```python
from build123d import *

# Parameters (mm, degrees)
SKETCH1_R           = 12.685
SKETCH1_R_2         = 3
BOSS_EXTRUDE1_DEPTH = 5
SKETCH2_R           = 6
SKETCH2_R_2         = 3
BOSS_EXTRUDE2_DEPTH = 9.25
SKETCH3_R           = 1.5
CUT_EXTRUDE1_DEPTH  = 12
SKETCH5_R           = 1.5
CUT_EXTRUDE3_DEPTH  = 21.183680289


with BuildPart() as part:
    # Sketch1 → Boss-Extrude1 (new body)
    with BuildSketch(Plane(origin=(0, 0, 0), x_dir=(1, 0, 0), z_dir=(0, 1, 0))):
        with Locations(Location((0, 0, 0), (0, 0, 270))):
            Circle(SKETCH1_R)
        with Locations(Location((0, 0, 0), (0, 0, 270))):
            Circle(SKETCH1_R_2, mode=Mode.SUBTRACT)
    extrude(amount=BOSS_EXTRUDE1_DEPTH)

    # Sketch2 → Boss-Extrude2 (add)
    with BuildSketch(Plane(origin=(0, 0, 0), x_dir=(1, 0, 0), z_dir=(0, 1, 0))):
        with Locations(Location((0, 0, 0), (0, 0, 270))):
            Circle(SKETCH2_R)
        with Locations(Location((0, 0, 0), (0, 0, 270))):
            Circle(SKETCH2_R_2, mode=Mode.SUBTRACT)
    extrude(amount=BOSS_EXTRUDE2_DEPTH)

    # Sketch3 → Cut-Extrude1 (cut)
    with BuildSketch(Plane(origin=(0, 0, 0), x_dir=(1, 0, 0), z_dir=(0, 1, 0))):
        with Locations(Location((0, 10, 0), (0, 0, 270))):
            Circle(SKETCH3_R)
        with Locations(Location((8.660254038, 5, 0), (0, 0, 270))):
            Circle(SKETCH3_R)
        with Locations(Location((8.660254038, -5, 0), (0, 0, 270))):
            Circle(SKETCH3_R)
        with Locations(Location((0, -10, 0), (0, 0, 270))):
            Circle(SKETCH3_R)
        with Locations(Location((-8.660254038, -5, 0), (0, 0, 270))):
            Circle(SKETCH3_R)
        with Locations(Location((-8.660254038, 5, 0), (0, 0, 270))):
            Circle(SKETCH3_R)
    extrude(amount=CUT_EXTRUDE1_DEPTH, mode=Mode.SUBTRACT)

    # Sketch5 → Cut-Extrude3 (cut, through all)
    with BuildSketch(Plane(origin=(0, 0, 0), x_dir=(0, -1, 0), z_dir=(1, 0, 0))):
        with Locations(Location((-6.75, 0, 0), (0, 0, 90))):
            Circle(SKETCH5_R)
        with Locations(Location((-2.5, 0, 0), (0, 0, 90))):
            Circle(SKETCH5_R)
    extrude(amount=-CUT_EXTRUDE3_DEPTH, mode=Mode.SUBTRACT)


solid = part.part
```
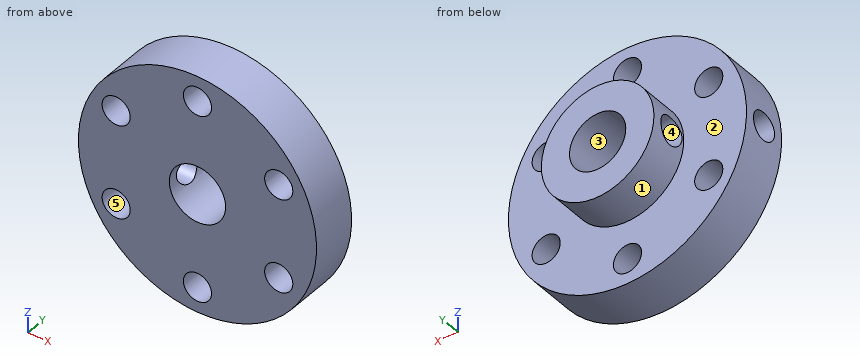
For this review, take the finished solid that the model builds, in its own axes (mm). Face numbers are marked on the shaded views. A direction names the side the tool comes from. Coordinates: 2 decimals unless noted, no trailing zeros. Order: outer loops, then holes, each group sorted by start corner. A loop starts at its lowest first (then second) coordinate and runs counter-clockwise, first axis right, second up. Notation, with made-up numbers: (43, 31) - (67, 31) arc R19 ccw to (67, 44) - close; hole circle Ø1 at (-7, -10). An arc over 180 degrees is marked (long way). Answer as a JSON object with one key per item and string values. Group by question number.
1. We need section B-B on z = 0. State the section outline as (x, y) points (3 decimals).
2. Clearance check with flat-ended pins moving along their axes: P1, Ø1.8, axis at y = 6.75, z = 0, coming from the -X side; P2, Ø1.8, axis at x = -8.66, z = 5, coming from the -Y side; P3, Ø3.5, axis at x = -8.66, z = -5, coming from the +Y side; P4, Ø5, axis at x = -4.5, y = 2, coming from the +Z side. State where each tip first meets the part, or that it passes through.
3. We need section D-D on z = 5.5. State the section outline as (x, y) points, then the cut area to 3 significant figures.
4. For probe 1 along Y at (x, z) = (-4.75, 0); probe 2 along Z at (x, y) = (-8.75, 3.5); probe 3 along X at (y, z) = (2.85, -5), list the stretches that pass through material, from the lowest coordinate up.
5. For the marked faces 4 and 5, list the 3-axis set-ups (+Z, -Z, +X, -X, +Y, -Y) from which the entire face can be reached by the end or side of a thin tool; tool diameter is ignored.
6. The part is to be moulded in two halves that separate along X. For the marked faces 1, 2 and 3, say which applies: pulls with the +X half, pulls with the -X half, needs draft (parallel to the pull), parting line crosses it, or undercut.
7. We need section A-A on x = 0. State the section outline as (y, z) points (3 decimals), then the cut area to 4 significant figures.
8. We need section C-C on x = -9. State the section outline as (y, z) points, then the cut area to 3 significant figures.
Final values:
{
 "1": {"outline": "(-12.685, 0) - (-3, 0) - (-3, 1) - (-12.685, 1) - close; (-12.685, 4) - (-3, 4) - (-3, 5.25) - (-6, 5.25) - (-6, 5) - (-12.685, 5) - close; (-6, 8.25) - (-3, 8.25) - (-3, 9.25) - (-6, 9.25) - close; (3, 0) - (12.685, 0) - (12.685, 5) - (6, 5) - (6, 9.25) - (3, 9.25) - close"},
 "2": {"P1": "x = 2.86", "P2": "through", "P3": "y = 5", "P4": "z = 12.53"},
 "3": {"outline": "(-11.43, 0) - (-10.07, 0) - (-10.07, 5) - (-11.43, 5) - close; (-7.25, 0) - (7.25, 0) - (7.25, 5) - (2.4, 5) - (2.4, 9.25) - (-2.4, 9.25) - (-2.4, 5) - (-7.25, 5) - close; (10.07, 0) - (11.43, 0) - (11.43, 5) - (10.07, 5) - close", "area": "106 mm²"},
 "4": {"probe 1": "0 to 1, 4 to 5.25, 8.25 to 9.25", "probe 2": "-9.18 to -6.5, -3.5 to -1.12, 1.12 to 3.5, 6.5 to 9.18", "probe 3": "-11.66 to -10.16, -7.16 to 7.16, 10.16 to 11.66"},
 "5": {"face 4": "-X", "face 5": "+Y, -Y"},
 "6": {"face 1": "parting line crosses it", "face 2": "needs draft", "face 3": "undercut"},
 "7": {"outline": "(0, -12.685) - (5, -12.685) - (5, -11.5) - (0, -11.5) - close; (0, -8.5) - (5, -8.5) - (5, -6) - (9.25, -6) - (9.25, -3) - (0, -3) - close; (0, 3) - (9.25, 3) - (9.25, 6) - (5, 6) - (5, 8.5) - (0, 8.5) - close; (0, 11.5) - (5, 11.5) - (5, 12.685) - (0, 12.685) - close", "area": "92.35 mm²"},
 "8": {"outline": "(0, -8.94) - (5, -8.94) - (5, -6.46) - (0, -6.46) - close; (0, -3.54) - (5, -3.54) - (5, 3.54) - (0, 3.54) - close; (0, 6.46) - (5, 6.46) - (5, 8.94) - (0, 8.94) - close; hole circle Ø3 at (2.5, 0)", "area": "53.1 mm²"}
}
